```python
from build123d import *

# Parameters (mm, degrees)
F0_R          = 1.5875
F1_DEPTH      = 1.5875
F1_DEPTH_BACK = 1.5875
F2_R          = 1.516292
F3_DEPTH      = 3.175
F3_DEPTH_BACK = 6.35
F4_W          = 11.43
F4_H          = 10.16
F5_DEPTH      = 3.175


with BuildPart() as f1:
    # F0 (on Front) → F1 (new body, two sides)
    with BuildSketch(Plane.XZ) as f1_sk:
        with BuildLine():
            Line((20.32, 5.08), (0, 5.08))
            ThreePointArc((0, 5.08), (-5.08, 0), (0, -5.08))
            Line((0, -5.08), (20.32, -5.08))
            ThreePointArc((20.32, -5.08), (25.4, 0), (20.32, 5.08))
        make_face()
        Circle(F0_R, mode=Mode.SUBTRACT)
        with Locations((20.32, 0)):
            Circle(F0_R, mode=Mode.SUBTRACT)
    extrude(amount=F1_DEPTH)
    extrude(f1_sk.sketch, amount=-F1_DEPTH_BACK)

    # F2 (on face) → F3 (join, two sides)
    with BuildSketch(Plane.XZ.offset(1.5875)) as f3_sk:
        with BuildLine():
            Line((7.141738, 5.08), (0, 5.08))
            ThreePointArc((0, 5.08), (-5.08, 0), (0, -5.08))
            Line((0, -5.08), (7.141738, -5.08))
            ThreePointArc((7.141738, -5.08), (12.221738, 0), (7.141738, 5.08))
        make_face()
        Circle(F2_R, mode=Mode.SUBTRACT)
    extrude(amount=F3_DEPTH)
    extrude(f3_sk.sketch, amount=-F3_DEPTH_BACK)

    # F4 (on face) → F5 (cut)
    with BuildSketch(Plane.XZ.offset(1.5875)):
        with Locations((-0.635, 0)):
            Rectangle(F4_W, F4_H)
    extrude(amount=-F5_DEPTH, mode=Mode.SUBTRACT)


solid = f1.part
```
CAD build for the part. Positions are in the model's coordinates, mm. A direction names the side the tool comes from. Coordinates: 2 decimals unless noted, no trailing zeros. Order: outer loops, then holes, each group sorted by start corner. A loop starts at its lowest first (then second) coordinate and runs counter-clockwise, first axis right, second up. Notation, with made-up numbers: M -16,72.5 L 28,72.5 A24 cw 28,98.5 Z; hole C 37.5,13 d2. An arc over 180 degrees is marked long. Write each question's results on one line, items separated by ' | '. Start each with the question number.
Q1. Which spindle directions (+Z, -Z, +X, -X, +Y, -Y) get a long thin tool onto all of the face, cutting with end or side? Do faces 1 (the flat face through (5.08, 0, 0)), 2 (the cylindrical face through (12.22, -3.15, -0.11)), 3 (the cylindrical face through (-1.203, 3.153, -0.923)). Say none if no direction does.
Q2. Drill centre lines: probe 1 along Y at (x, z) = (-2, 4.5); probe 2 along Z at (x, y) = (20.32, -0.3); probe 3 along Y at (x, z) = (12.5, 2.75). Where is each one in solid material? Low to high. Write a range as from..to.
Q3. Pull direction X, two halves, no side cores. Call faces 4 (the cylindrical face through (-5.08, 3.2, 0.11)), 5 (the cylindrical face through (12.22, 3.15, -0.11)), 6 (the cylindrical face through (18.734, 0.022, 0.07)): +X half, -X half, draft (parallel to the pull), parting line (faces both ways), or undercut.
Q4. Cut at B-B (y = 1). List the corners of the cut face in (x, z) (1 decimal).
Q5. Cut at A-A (x = 3). List the corners of the cut face in (y, z).
Q6. Cut at C-C (z = 0). List the corners of the cut face in (x, y), then the cut area to 3 significant figures.
Q7. Cut at D-D (z = -2.5). List the corners of the cut face in (x, y), then the cut area to 3 significant figures.
Q8. Flat gauge pins, fed straight in: P1, Ø1.9, axis at x = 20.32, z = 0, coming from the -Y side; P2, Ø1.5, axis at x = 18, z = -0.5, coming from the +Y side; P3, Ø3, axis at y = -2.5, z = 3, coming from the +X side; P4, Ø3, axis at y = 1, z = 1.5, coming from the -X side. Where does each tip first touch, or does it go through?
Found:
1) face 1: +Z, -Z, -X | face 2: +X, -Y | face 3: +Y, -Y
2) probe 1: -4.76..-1.59, 1.59..4.76 | probe 2: -5.08..-1.59, 1.59..5.08 | probe 3: -1.59..1.59
3) face 4: -X half | face 5: +X half | face 6: undercut
4) outline: M 5.1,-5.1 L 20.3,-5.1 A5.1 ccw 20.3,5.1 L 5.1,5.1 Z; hole C 20.3,0 d3.2
5) outline: M -4.76,-5.08 L -1.59,-5.08 L -1.59,5.08 L -4.76,5.08 Z; M 1.59,-5.08 L 4.76,-5.08 L 4.76,5.08 L 1.59,5.08 Z
6) outline: M -5.08,-4.76 L -1.52,-4.76 L -1.52,-1.59 L -5.08,-1.59 Z; M -5.08,1.59 L -1.52,1.59 L -1.52,4.76 L -5.08,4.76 Z; M 1.52,-4.76 L 12.22,-4.76 L 12.22,-1.59 L 18.73,-1.59 L 18.73,1.59 L 12.22,1.59 L 12.22,4.76 L 1.52,4.76 L 1.52,1.59 L 5.08,1.59 L 5.08,-1.59 L 1.52,-1.59 Z; M 21.91,-1.59 L 25.4,-1.59 L 25.4,1.59 L 21.91,1.59 Z | area: 145 mm²
7) outline: M -4.42,-4.76 L 11.56,-4.76 L 11.56,-1.59 L 24.74,-1.59 L 24.74,1.59 L 11.56,1.59 L 11.56,4.76 L -4.42,4.76 L -4.42,1.59 L 5.08,1.59 L 5.08,-1.59 L -4.42,-1.59 Z | area: 164 mm²
8) P1: through | P2: y = 1.59 | P3: x = 25.07 | P4: x = -5.08
